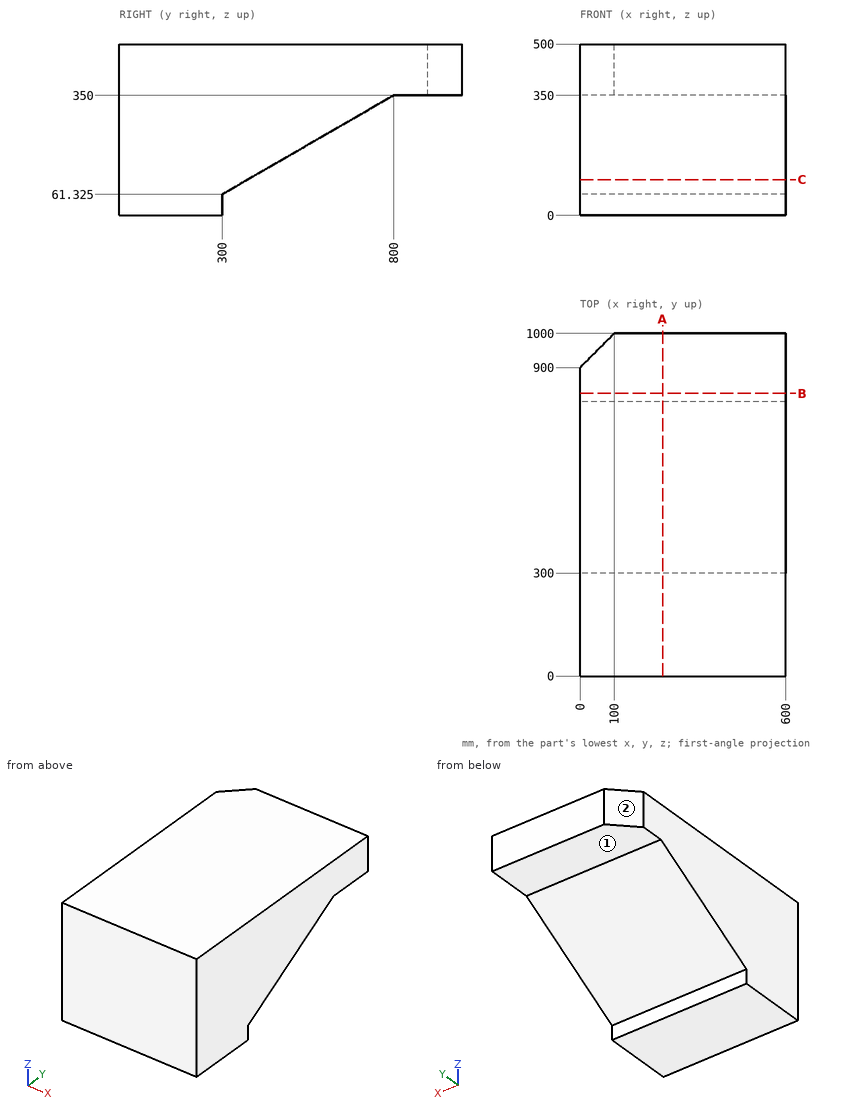
Geometry: see drawing. Coordinates: mm, zero at the bounding-box minimum. A direction names the side the tool comes from. Give positions to 0.01 mm unless a question says otherwise; leave off trailing zeros. Order: outer loops, then holes, each group sorted by start corner. A loop starts at its lowest first (then second) coordinate and runs counter-clockwise, first axis right, second up. Notation, with made-up numbers: (-17.75, -3) - (-10.75, -3) arc R25 cw to (-10.75, 13) - close; hole circle Ø2 at (-1.5, -21.5). An arc over 180 degrees is marked (long way). Write each question's results on one line, items separated by ' | '.
Item 1: Section B-B (y = 825). Return loops of the section in (x, z).
A:
outline: (0, 350) - (600, 350) - (600, 500) - (0, 500) - close
Item 2: Section C-C (z = 104.5). Return loops of the section in (x, y).
A:
outline: (0, 0) - (600, 0) - (600, 374.78) - (0, 374.78) - close
Item 3: Access query for the marked faces 1 and 2. Directions: +Z, -Z, +X, -X, +Y, -Y. A direction counts if a zero-diameter tool reaches every point of the face in a straight line with its end or side. Return the directions, or none.
A:
face 1: -Z, +X, -X, +Y | face 2: +Z, -Z, -X, +Y
Item 4: Section A-A (x = 241). Return loops of the section in (y, z) (3 decimals).
A:
outline: (0, 0) - (300, 0) - (300, 61.325) - (800, 350) - (1000, 350) - (1000, 500) - (0, 500) - close
Item 5: Material intervals for line 1 along Z through (x, y) = (491.5, 810.5); line 2 along Y through (x, z) = (436, 286); line 3 along Z through (x, y) = (548.5, 764.5), sorted ascending.
A:
line 1: z = 350 to 500 | line 2: y = 0 to 689.15 | line 3: z = 329.5 to 500
Item 6: Contact query for a flat-ended pin moving along its axis: pin 1 Ø3 at (x, y) = (273, 492) entering from -Z. Output: stop coordinate, or through.
A:
pin 1: stops at z = 171.31
